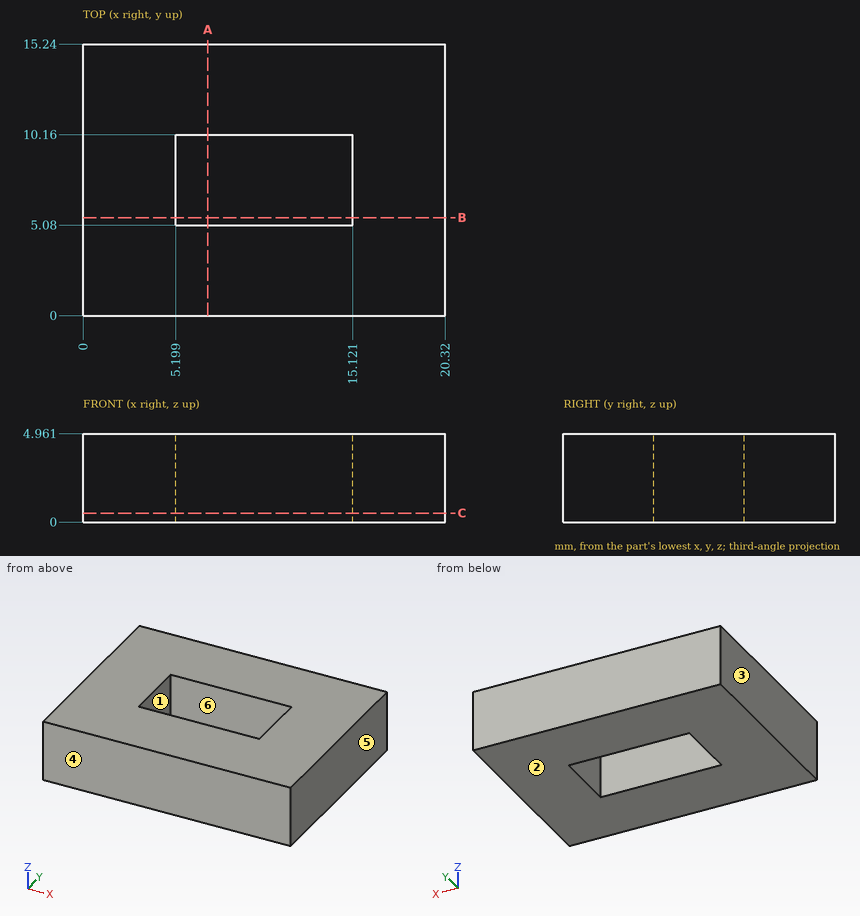
Study the drawing (mm; zero at the part's minimum x, y, z) and answer. A direction names the side the tool comes from. Coordinates: 2 decimals unless noted, no trailing zeros. Write each loop counter-clockwise with the first axis right and the second up, starting at its lowest first coordinate (ties: lowest second). Pieces come first, ordered by that corner, then holes. Notation, with made-up numbers: (-39, -2.5) - (-27, -2.5) arc R26 cw to (-27, 12.5) - close; hole circle Ø2 at (55, 83). An arc over 180 degrees is marked (long way). One line per question, with ' | ' between items.
1) Find section C-C, the plane z = 0.5. Determine the outline of the cut face in (x, y), and give its area (3 significant figures).
Checks:
outline: (0, 0) - (20.32, 0) - (20.32, 15.24) - (0, 15.24) - close; hole (5.2, 5.08) - (15.12, 5.08) - (15.12, 10.16) - (5.2, 10.16) - close | area: 259 mm2
2) Consider probe 1 along X at (y, z) = (8, 4.25); probe 2 along Y at (x, z) = (7.75, 2.4). Determine where each line is inside the solid, lowest interval first. Write a range as [from, to].
Checks:
probe 1: [0, 5.2], [15.12, 20.32] | probe 2: [0, 5.08], [10.16, 15.24]
3) For the marked faces 1 and 2, determine the directions among +Z, -Z, +X, -X, +Y, -Y from which every point of the face is accessible in a straight line to the end or side of a thin tool.
Checks:
face 1: +Z, -Z | face 2: -Z, +X, -X, +Y, -Y
4) Find section B-B, the plane y = 5.5. Determine the outline of the cut face in (x, z), and give its area (3 significant figures).
Checks:
outline: (0, 0) - (5.2, 0) - (5.2, 4.96) - (0, 4.96) - close; (15.12, 0) - (20.32, 0) - (20.32, 4.96) - (15.12, 4.96) - close | area: 51.6 mm2
5) Find section A-A, the plane x = 7. Determine the outline of the cut face in (y, z).
Checks:
outline: (0, 0) - (5.08, 0) - (5.08, 4.96) - (0, 4.96) - close; (10.16, 0) - (15.24, 0) - (15.24, 4.96) - (10.16, 4.96) - close
6) The mould has two halves that part along X. Classify the marked faces 3, 4, 5 and 6: +X half, -X half, draft (parallel to the pull), parting line (faces both ways), or undercut.
Checks:
face 3: -X half | face 4: draft | face 5: +X half | face 6: undercut
